Design review of the part shown in the three views and the two pictorial views. Dimensions are in mm from the part's minimum x, y and z. Coordinates: 2 decimals unless noted, no trailing zeros. Write each loop counter-clockwise with the first axis right and the second up, starting at its lowest first coordinate (ties: lowest second). Pieces come first, ordered by that corner, then holes. Notation, with made-up numbers: (82, 16) - (100, 16) arc R18 cw to (100, 50) - close; hole circle Ø2 at (-17, 64). An arc over 180 degrees is marked (long way). Return JSON: item names as keys, results as strings. Group by question number.
(1) We need section B-B on x = 19. State the section outline as (y, z) points (3 decimals), then the cut area to 3 significant figures.
(2) We need section A-A on y = 1.35. State the section outline as (x, z) points (3 decimals), then the cut area to 3 significant figures.
(3) We need section C-C on z = 11.25. State the section outline as (x, y) points (3 decimals).
(4) To check wall thickness, follow L1, parallel to X at y = 1.45, z = 21.75; L2, parallel to X at y = 2.65, z = 9.25 (3 decimals); L3, parallel to Z at x = 20, y = 1.05 (3 decimals). State the ranges of each line that lie inside material, in increasing order. Write a range as from..to.
(5) For pin 1 Ø3 at (x, z) = (29.5, 20) entering from -Y; pin 2 Ø1.6 at (x, y) = (42, 1) entering from +Z; pin 3 Ø1.6 at (x, y) = (42, 2) entering from -Z (3 decimals), all flat-tipped, find the tip position at first contact; note any pin that passes through.
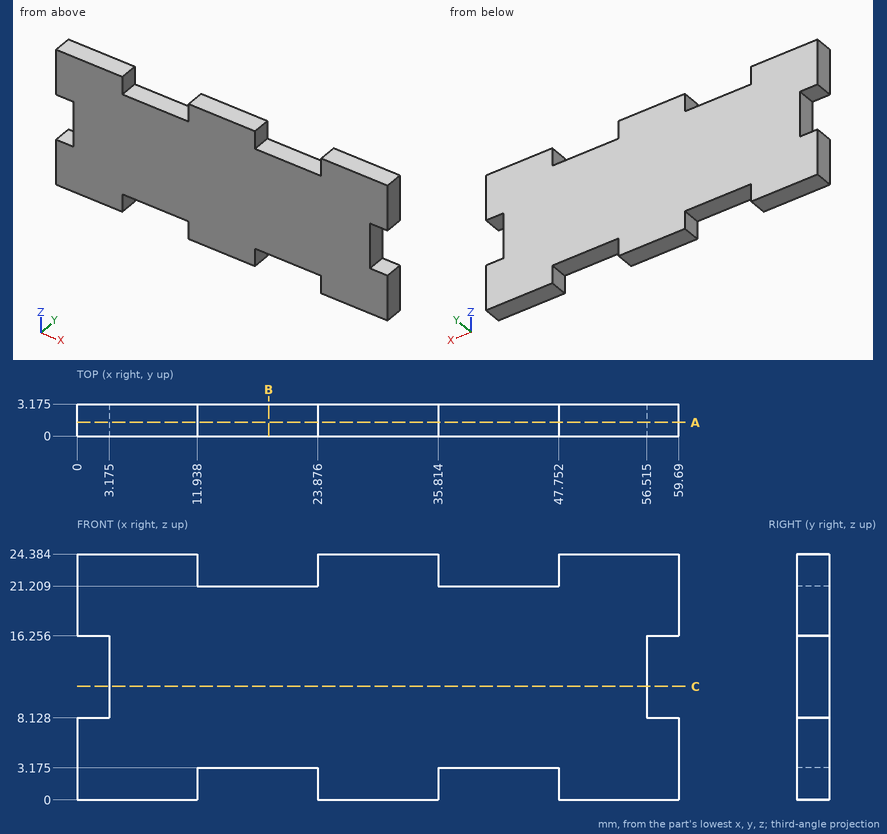
Ans:
{
 "1": {"outline": "(0, 3.175) - (3.175, 3.175) - (3.175, 21.209) - (0, 21.209) - close", "area": "57.3 mm²"},
 "2": {"outline": "(0, 0) - (11.938, 0) - (11.938, 3.175) - (23.876, 3.175) - (23.876, 0) - (35.814, 0) - (35.814, 3.175) - (47.752, 3.175) - (47.752, 0) - (59.69, 0) - (59.69, 8.128) - (56.515, 8.128) - (56.515, 16.256) - (59.69, 16.256) - (59.69, 24.384) - (47.752, 24.384) - (47.752, 21.209) - (35.814, 21.209) - (35.814, 24.384) - (23.876, 24.384) - (23.876, 21.209) - (11.938, 21.209) - (11.938, 24.384) - (0, 24.384) - (0, 16.256) - (3.175, 16.256) - (3.175, 8.128) - (0, 8.128) - close", "area": "1,250 mm²"},
 "3": {"outline": "(3.175, 0) - (56.515, 0) - (56.515, 3.175) - (3.175, 3.175) - close"},
 "4": {"L1": "0..11.94, 23.88..35.81, 47.75..59.69", "L2": "3.175..56.515", "L3": "3.175..21.209"},
 "5": {"pin 1": "y = 0", "pin 2": "z = 21.21", "pin 3": "z = 3.175"}
}
